Check sheet for the modelled part. Datum: model origin and axes. Units: mm. Face numbers are marked on the shaded views. A direction names the side the tool comes from. Give positions to 0.01 mm unless a question says otherwise; leave off trailing zeros. Write each loop counter-clockwise with the first axis right and the second up, starting at its lowest first coordinate (ties: lowest second). Pieces come first, ordered by that corner, then holes. Notation, with made-up numbers: M 71,35.5 L 96,35.5 A17 ccw 96,65.5 Z; hole C -13.75,-20.75 d1. An arc over 180 degrees is marked long. Use CSV: the item, a comma, the result in double quotes. Start each with the question number.
1. Mould release check, pull along X, two halves, no side actions. Record for the marked faces 1, 2 and 3: +X half, -X half, draft (parallel to the pull), parting line (faces both ways), or undercut.
2. Scan lines: line 1 (X direction, y = -15.45, z = 9.5); line 2 (Z direction, x = 35.5, y = -8); line 3 (Y direction, x = 40.5, z = 2.75). Record each from-to range of solid material in increasing order.
3. Cross-section at D-D, the plane z = 3. Enter the section's corners in (x, y), and give its area (3 significant figures).
4. Cross-section at A-A, the plane y = 17. Enter the section's corners in (x, z), and give its area (3 significant figures).
5. Cross-section at B-B, the plane z = 21. Enter the section's corners in (x, y).
6. Depth check by flat-ended pin: P1, Ø3.5, axis at x = 6.76, z = 16, coming from the -Y side; P2, Ø5, axis at x = -5.42, z = 15.18, coming from the +Y side; P3, Ø8, axis at y = 3, z = 11.5, coming from the +X side; P4, Ø4.5, axis at y = 4, z = 7, coming from the +X side. Enter the tip coordinate at first touch or a pass-through.
7. Cross-section at C-C, the plane x = 26.5. Enter the section's corners in (y, z), and give its area (3 significant figures).
8. Access from +Z, -Z, +X, -X, +Y, -Y to the whole of each face (thin tool, end or side, straight path). Record for the marked faces 4 and 5.
from build123d import *

# Parameters (mm, degrees)
SKETCH1_W           = 57.5
SKETCH1_H           = 45
BOSS_EXTRUDE1_DEPTH = 4
SKETCH4_W           = 24
SKETCH4_H           = 4
BOSS_EXTRUDE4_DEPTH = 24
CUT_EXTRUDE1_START  = -4
CUT_EXTRUDE1_DEPTH  = 4
SKETCH6_R           = 3
SKETCH6_R_2         = 2
CUT_EXTRUDE2_DEPTH  = 24
SKETCH7_R           = 2
SKETCH7_W           = 40
SKETCH7_H           = 20
CUT_EXTRUDE3_DEPTH  = 24
FILLET2_R           = 5
SKETCH9_W           = 40
SKETCH9_H           = 2
BOSS_EXTRUDE5_DEPTH = 4
RIB1_REACH          = 61.005
SKETCH10_WALL_W     = 125.416867366
SKETCH10_WALL_H     = 2
RIB5_REACH          = 61.005
SKETCH11_WALL_W     = 125.5713139
SKETCH11_WALL_H     = 2
SKETCH13_W          = 12
SKETCH13_H          = 4
BOSS_EXTRUDE7_DEPTH = 4
SKETCH15_W          = 4
SKETCH15_H          = 12
BOSS_EXTRUDE8_DEPTH = 19
CUT_EXTRUDE4_DEPTH  = 15
FILLET5_R           = 5
FILLET6_R           = 5


# Read off the part's stored shape, not the designer's step: Cut-Extrude1
with BuildPart() as part:
    # Sketch1 → Boss-Extrude1 (new body)
    with BuildSketch(Plane.XY):
        with Locations((17.830298358, 6.093256958)):
            Rectangle(SKETCH1_W, SKETCH1_H)
    extrude(amount=BOSS_EXTRUDE1_DEPTH)

    # Sketch4 → Boss-Extrude4 (add)
    with BuildSketch(Plane.XY.offset(4)):
        with Locations((1.080298358, -14.406743042)):
            Rectangle(SKETCH4_W, SKETCH4_H)
    extrude(amount=BOSS_EXTRUDE4_DEPTH)

    # Cut-Extrude1 outline → Cut-Extrude1 (cut)
    with BuildSketch(Plane(origin=(0, -12.406743042, 0), x_dir=(1, 0, 0), z_dir=(0, 1, 0)).offset(CUT_EXTRUDE1_START)):
        with BuildLine():
            Line((13.080298358, -28), (13.080298358, -16))
            ThreePointArc((13.080298358, -16), (9.565579732, -24.485281374), (1.080298358, -28))
            Line((1.080298358, -28), (13.080298358, -28))
        make_face()
        with BuildLine():
            Line((-10.919701642, -28), (1.080298358, -28))
            ThreePointArc((1.080298358, -28), (-7.404983016, -24.485281374), (-10.919701642, -16))
            Line((-10.919701642, -16), (-10.919701642, -28))
        make_face()
    extrude(amount=CUT_EXTRUDE1_DEPTH, mode=Mode.SUBTRACT)

    # Sketch6 → Cut-Extrude2 (cut)
    with BuildSketch(Plane(origin=(0, -12.406743042, 0), x_dir=(1, 0, 0), z_dir=(0, 1, 0))):
        with Locations(Location((1.080298358, -16, 0), (0, 0, 270))):
            Circle(SKETCH6_R)
        with Locations(Location((1.080298358, -9.5, 0), (0, 0, 270))):
            Circle(SKETCH6_R_2)
        with Locations(Location((6.762193148, -16, 0), (0, 0, 270))):
            Circle(SKETCH6_R_2)
        with Locations(Location((0.262193148, -21.681894789, 0), (0, 0, 270))):
            Circle(SKETCH6_R_2)
        with Locations(Location((-5.419701642, -15.181894789, 0), (0, 0, 270))):
            Circle(SKETCH6_R_2)
    extrude(amount=-CUT_EXTRUDE2_DEPTH, mode=Mode.SUBTRACT)

    # Sketch7 → Cut-Extrude3 (cut)
    with BuildSketch(Plane.XY.offset(4)):
        with Locations((-5.919701642, 23.593256958)):
            Circle(SKETCH7_R)
        with Locations((-5.919701642, 13.593256958)):
            Circle(SKETCH7_R)
        with Locations((41.580298358, 23.593256958)):
            Circle(SKETCH7_R)
        with Locations((41.580298358, 13.593256958)):
            Circle(SKETCH7_R)
        with Locations((17.830298358, 18.593256958)):
            Rectangle(SKETCH7_W, SKETCH7_H)
    extrude(amount=-CUT_EXTRUDE3_DEPTH, mode=Mode.SUBTRACT)

    # Fillet2
    fillet2_edges = [part.edges().sort_by_distance(p)[0] for p in [
        (-10.919701642, 28.593256958, 2),
        (46.580298358, 28.593256958, 2),
    ]]
    fillet(fillet2_edges, radius=FILLET2_R)

    # Sketch9 → Boss-Extrude5 (add)
    with BuildSketch(Plane.XY.offset(4)):
        with Locations((17.830298358, 7.593256958)):
            Rectangle(SKETCH9_W, SKETCH9_H)
    extrude(amount=BOSS_EXTRUDE5_DEPTH)

    # Sketch10 wall → Rib1 (add, up to next)
    with BuildSketch(Plane(origin=(37.830298358, 4.600713915, 6.172546288), x_dir=(0, -0.736977999751, -0.675916731471), z_dir=(0, 0.675916731471, -0.736977999751)), mode=Mode.PRIVATE) as rib1_sk1:
        with Locations((0, 1)):
            Rectangle(SKETCH10_WALL_W, SKETCH10_WALL_H)
    rib1_tool1 = extrude(rib1_sk1.sketch, amount=RIB1_REACH, mode=Mode.PRIVATE) - part.part
    add(rib1_tool1.solids().sort_by_distance((37.830298358, 4.600713915, 6.172546288))[0])

    # Sketch11 wall → Rib5 (add, up to next)
    with BuildSketch(Plane(origin=(-2.169701642, 4.593256958, 6.067812051), x_dir=(0, -0.719194164668, -0.694809148981), z_dir=(0, 0.694809148981, -0.719194164668)), mode=Mode.PRIVATE) as rib5_sk1:
        with Locations((0, -1)):
            Rectangle(SKETCH11_WALL_W, SKETCH11_WALL_H)
    rib5_tool1 = extrude(rib5_sk1.sketch, amount=RIB5_REACH, mode=Mode.PRIVATE) - part.part
    add(rib5_tool1.solids().sort_by_distance((-2.169701642, 4.593256958, 6.067812051))[0])

    # Sketch13 → Boss-Extrude7 (add)
    with BuildSketch(Plane(origin=(13.080298358, 0, 0), x_dir=(0, 0, -1), z_dir=(1, 0, 0))):
        with Locations((-10, -14.406743042)):
            Rectangle(SKETCH13_W, SKETCH13_H)
    extrude(amount=BOSS_EXTRUDE7_DEPTH)

    # Sketch15 → Boss-Extrude8 (add)
    with BuildSketch(Plane(origin=(0, -12.406743042, 0), x_dir=(1, 0, 0), z_dir=(0, 1, 0))):
        with Locations((15.080298358, -10)):
            Rectangle(SKETCH15_W, SKETCH15_H)
    extrude(amount=BOSS_EXTRUDE8_DEPTH)

    # Sketch16 → Cut-Extrude4 (cut)
    with BuildSketch(Plane.ZY.offset(-13.080298358)):
        Polygon((8, 6.593256958), (8, -3.406743042), (16, -12.406743042), (16, 6.593256958), align=None)
    extrude(amount=-CUT_EXTRUDE4_DEPTH, mode=Mode.SUBTRACT)

    # Fillet5
    # the kernel refuses this fillet: 5 mm, written as the material it adds along each edge
    with BuildSketch(Plane(origin=(13.080298358, -16.406743042, 16), x_dir=(1, 0, 0), z_dir=(0, 1, 0))) as fillet5_piece_1:
        with BuildLine():
            CenterArc((4.25, -4.993746089), FILLET5_R, 92.865983979, 70.051432775)
            ThreePointArc((-0.529411765, -3.524997239), (-0.133090992, -1.782265577), (0, 0))
            Line((0, 0), (4, 0))
        make_face()
    extrude(amount=4)

    # Fillet6
    fillet6_edges = [part.edges().sort_by_distance(p)[0] for p in [
        (17.080298358, 6.593256958, 6),
        (13.080298358, 6.593256958, 6),
        (15.080298358, -3.406743042, 8),
        (15.080298358, -12.406743042, 16),
    ]]
    fillet(fillet6_edges, radius=FILLET6_R)


solid = part.part
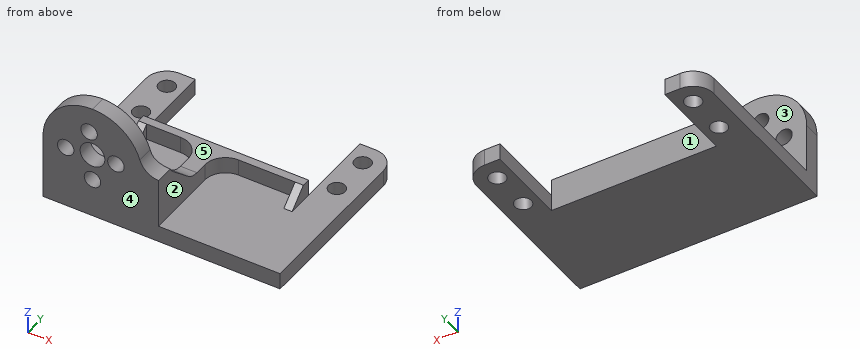
Worked answers:
1,face 1,"undercut"
1,face 2,"+X half"
1,face 3,"draft"
2,line 1,"x = -10.92 to -0.92, 3.08 to 17.08"
2,line 2,"z = 0 to 4"
2,line 3,"y = -16.41 to 11.91, 15.28 to 21.91, 25.28 to 28.59"
3,outline,"M -10.92,-16.41 L 46.58,-16.41 L 46.58,23.59 A5 ccw 41.58,28.59 L 37.83,28.59 L 37.83,8.59 L -2.17,8.59 L -2.17,28.59 L -5.92,28.59 A5 ccw -10.92,23.59 Z; hole C -5.92,13.59 d4; hole C -5.92,23.59 d4; hole C 41.58,13.59 d4; hole C 41.58,23.59 d4"
3,area,"1,730 mm^2"
4,outline,"M -10.92,0 L -2.17,0 L -2.17,4 L -10.92,4 Z; M 37.83,0 L 46.58,0 L 46.58,4 L 37.83,4 Z"
4,area,"70.0 mm^2"
5,outline,"M -9.83,-16.41 L -1.62,-16.41 L -1.62,-12.41 L -9.83,-12.41 Z; M 2.14,-16.41 L 11.99,-16.41 L 11.99,-12.41 L 2.14,-12.41 Z"
6,P1,"passes through"
6,P2,"stops at y = -12.41"
6,P3,"stops at x = 18.36"
6,P4,"stops at x = 37.83"
7,outline,"M -16.41,0 L 8.59,0 L 8.59,8 L 6.59,8 L 6.59,4 L -16.41,4 Z"
7,area,"108 mm^2"
8,face 4,"+Z, -Z, +X, -X, -Y"
8,face 5,"+Z, +X, -X, +Y"
